```python
from build123d import *

# Parameters (mm, degrees)
SKETCH1_R           = 2
SKETCH1_R_2         = 5.125
BOSS_EXTRUDE2_DEPTH = 3
SKETCH2_R           = 2
BOSS_EXTRUDE3_DEPTH = 3.5
BOSS_EXTRUDE4_START = -3
SKETCH3_R           = 12
SKETCH3_R_2         = 11.1
BOSS_EXTRUDE4_DEPTH = 3
FILLET1_R           = 30


with BuildPart() as part:
    # Sketch1 → Boss-Extrude2 (new body)
    with BuildSketch(Plane(origin=(0, 0, 0), x_dir=(1, 0, 0), z_dir=(0, 1, 0))):
        with BuildLine():
            Line((0, 11.1), (17.140916293, 11.1))
            ThreePointArc((17.140916293, 11.1), (20.836434423, 8.630733729), (19.969343418, 4.271572875))
            Line((19.969343418, 4.271572875), (-4.271572875, -19.969343418))
            ThreePointArc((-4.271572875, -19.969343418), (-8.630733729, -20.836434423), (-11.1, -17.140916293))
            Line((-11.1, -17.140916293), (-11.1, 0))
            ThreePointArc((-11.1, 0), (-7.848885271, 7.848885271), (0, 11.1))
        make_face()
        with Locations(Location((17.140916293, 7.1, 0), (0, 0, 270))):
            Circle(SKETCH1_R, mode=Mode.SUBTRACT)
        with Locations(Location((-7.1, -17.140916293, 0), (0, 0, 270))):
            Circle(SKETCH1_R, mode=Mode.SUBTRACT)
        with Locations(Location((0, 0, 0), (0, 0, 270))):
            Circle(SKETCH1_R_2, mode=Mode.SUBTRACT)
    extrude(amount=BOSS_EXTRUDE2_DEPTH)

    # Sketch2 → Boss-Extrude3 (add)
    with BuildSketch(Plane(origin=(0, 3, 0), x_dir=(1, 0, 0), z_dir=(0, 1, 0))):
        with Locations(Location((0, -8.1, 0), (0, 0, 270))):
            Circle(SKETCH2_R)
        with Locations(Location((0, 8.1, 0), (0, 0, 90))):
            Circle(SKETCH2_R)
        with Locations(Location((8.1, 0, 0), (0, 0, 90))):
            Circle(SKETCH2_R)
        with Locations(Location((-8.1, 0, 0), (0, 0, 270))):
            Circle(SKETCH2_R)
    extrude(amount=BOSS_EXTRUDE3_DEPTH)

    # Sketch3 → Boss-Extrude4 (add)
    with BuildSketch(Plane(origin=(0, 3, 0), x_dir=(1, 0, 0), z_dir=(0, 1, 0)).offset(BOSS_EXTRUDE4_START)):
        Circle(SKETCH3_R)
        Circle(SKETCH3_R_2, mode=Mode.SUBTRACT)
    extrude(amount=BOSS_EXTRUDE4_DEPTH)

    # Fillet1
    fillet1_edges = [part.edges().sort_by_distance(p)[0] for p in [
        (4.559605246, 1.5, -11.1),
        (-11.1, 1.5, 4.559605246),
        (4.624757482, 1.5, 11.07301306),
        (11.07301306, 1.5, 4.624757482),
    ]]
    fillet(fillet1_edges, radius=FILLET1_R)


solid = part.part
```
Verification items for the finished model (mm, model axes). A direction names the side the tool comes from. Round coordinates to 2 decimals unless told otherwise and drop trailing zeros. Write each loop counter-clockwise with the first axis right and the second up, starting at its lowest first coordinate (ties: lowest second). Pieces come first, ordered by that corner, then holes. Notation, with made-up numbers: (-6, 6.25) - (5, 6.25) arc R17 ccw to (5, 17.25) - close; hole circle Ø6 at (85.5, 50). An arc over 180 degrees is marked (long way). Answer as a JSON object with one key per item and string values. Group by question number.
Q1. Tool access check on faces 1 (the flat face through (-11.1, 1, 13)), 2 (the flat face through (8, 6.5, 0)), 3 (the cylindrical face through (1.2, 4.7, -6.5)). Record the directions out of +Z, -Z, +X, -X, +Y, -Y that give a thin tool (end or side, any length) a straight path to the whole face; none if there is none.
Q2. Thickness scan on line 1 (Y direction, x = 5, z = 6.5); line 2 (Z direction, x = 17, y = 2.5); line 3 (X direction, y = 1, z = 0) (3 decimals). Record the ranges inside material, lowest first.
Q3. Go/stop test with flat-tipped pins: pin 1 Ø12 at (x, z) = (0, 0) entering from +Y; pin 2 Ø2.5 at (y, z) = (2, 15) entering from -X; pin 3 Ø1.5 at (y, z) = (5, -8) entering from +X. Record where each tip stops, or that it passes through.
Q4. Section check A-A, the plane x = -3.5. Enter the section's corners in (y, z), plus the area to 3 significant figures.
Q5. Section check C-C, the plane y = 0.75. Enter the section's corners in (x, z) (3 decimals), plus the area to 3 significant figures.
Q6. Section check B-B, the plane z = 16.5. Enter the section's corners in (x, y).
Q7. Section check D-D, the plane x = 0. Enter the section's corners in (y, z) (3 decimals), plus the area to 3 significant figures.
Q8. Mould release check, pull along X, two halves, no side actions. Record for faces 4 (the flat face through (13, 1, -11.1)), 5 (the cylindrical face through (-8.012, 4.726, -1.998)), 6 (the cylindrical face through (8.46, 1.48, 8.51)), 7 (the cylindrical face through (8.012, 4.726, 1.998)): released by +X, released by -X, zero draft, split by the parting line, or undercut.
Found:
{
 "1": {"face 1": "+Z, -X, +Y, -Y", "face 2": "+Z, -Z, +X, -X, +Y", "face 3": "+Y"},
 "2": {"line 1": "y = 0 to 3", "line 2": "z = -11.1 to -9.1, -5.1 to -1.3", "line 3": "x = -12 to -5.125, 5.125 to 15.698"},
 "3": {"pin 1": "stops at y = 3", "pin 2": "stops at x = -11.1", "pin 3": "stops at x = 2"},
 "4": {"outline": "(0, -11.48) - (3, -11.48) - (3, -3.74) - (0, -3.74) - close; (0, 3.74) - (3, 3.74) - (3, 19.2) - (0, 19.2) - close", "area": "69.6 mm^2"},
 "5": {"outline": "(-11.743, 2.471) arc R12 ccw to (2.471, -11.743) arc R30 cw to (8.648, -11.1) - (17.141, -11.1) arc R4 ccw to (19.969, -4.272) - (13.964, 1.734) arc R30 cw to (10.051, 6.556) arc R12 ccw to (6.556, 10.051) arc R30 cw to (1.734, 13.964) - (-4.272, 19.969) arc R4 ccw to (-11.1, 17.141) - (-11.1, 8.648) arc R30 cw to start; hole circle Ø4 at (-7.1, 17.141); hole circle Ø10.25 at (0, 0); hole circle Ø4 at (17.141, -7.1)", "area": "574 mm^2"},
 "6": {"outline": "(-11.1, 0) - (-8.99, 0) - (-8.99, 3) - (-11.1, 3) - close; (-5.21, 0) - (-0.8, 0) - (-0.8, 3) - (-5.21, 3) - close"},
 "7": {"outline": "(0, -12) - (3, -12) - (3, -10.1) - (6.5, -10.1) - (6.5, -6.1) - (3, -6.1) - (3, -5.125) - (0, -5.125) - close; (0, 5.125) - (3, 5.125) - (3, 6.1) - (6.5, 6.1) - (6.5, 10.1) - (3, 10.1) - (3, 15.698) - (0, 15.698) - close", "area": "80.3 mm^2"},
 "8": {"face 4": "zero draft", "face 5": "undercut", "face 6": "released by +X", "face 7": "undercut"}
}
